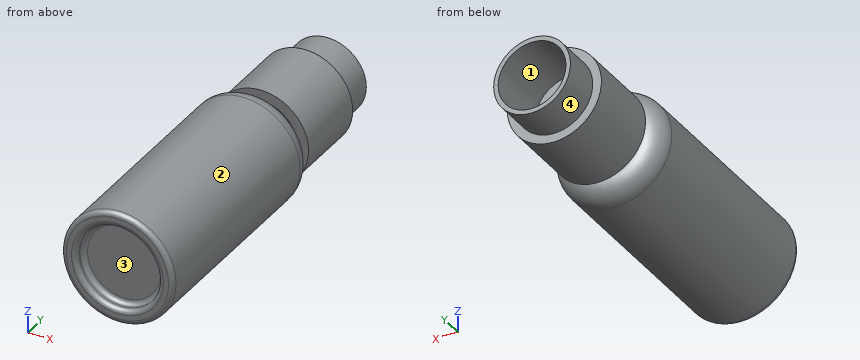
```python
from build123d import *


with BuildPart() as part:
    # Sketch1 → Revolve1 (revolve)
    with BuildSketch(Plane.XY):
        with BuildLine():
            ThreePointArc((8.75, 1), (9.042893219, 0.292893219), (9.75, 0))
            Line((9.75, 0), (10.875, 0))
            ThreePointArc((10.875, 0), (11.582106781, 0.292893219), (11.875, 1))
            Line((11.875, 1), (11.875, 46.5))
            ThreePointArc((11.875, 46.5), (10.593592168, 49.593592168), (7.5, 50.875))
            Line((7.5, 50.875), (7.75, 50.875))
            Line((7.75, 50.875), (7.75, 52.875))
            Line((7.75, 52.875), (10, 52.875))
            Line((10, 52.875), (10, 69.075))
            Line((10, 69.075), (8.15, 69.075))
            Line((8.15, 69.075), (8.15, 77.275))
            Line((8.15, 77.275), (7.2, 77.275))
            Line((7.2, 77.275), (7.2, 63.575))
            Line((7.2, 63.575), (0, 63.575))
            Line((0, 63.575), (0, 2.409558552))
            Line((0, 2.409558552), (7.75, 2.409558552))
            ThreePointArc((7.75, 2.409558552), (8.457106781, 2.116665333), (8.75, 1.409558552))
            Line((8.75, 1.409558552), (8.75, 1))
        make_face()
    revolve(axis=Axis((0, 65.8, 0), (0, -1, 0)))


solid = part.part
```
Geometry: final body of the model. Coordinates: model frame, mm. Face numbers are marked on the shaded views. A direction names the side the tool comes from. Coordinates: 2 decimals unless noted, no trailing zeros. Order: outer loops, then holes, each group sorted by start corner. A loop starts at its lowest first (then second) coordinate and runs counter-clockwise, first axis right, second up. Notation, with made-up numbers: M 9.25,45 L 26.25,45 A17 ccw 26.25,71 Z; hole C -14.75,12 d4. An arc over 180 degrees is marked long. Answer in a Markdown table with one row per item. Add a question column.
Q1. Reachability of the marked faces 1 and 2 from +Z, -Z, +X, -X, +Y, -Y: full face, straight path, thin tool, end or side. Return the list, or none.
Q2. Section query C-C on y = 18. Return the cut outline in (x, z) (3 decimals).
Q3. Mould query, pull axis X, two halves, no side actions, for the marked faces 3 and 4. Classes: released by +X, released by -X, zero draft, split by the parting line, or undercut.
Q4. Contact query for flat-ended pins moving along their axis: P1, Ø6, axis at x = -4.5, z = -4, coming from the -Y side; P2, Ø4, axis at x = 6, y = 45, coming from the +Z side; P3, Ø4, axis at x = 7, y = 14, coming from the -Z side. Output: stop coordinate, or through.
Q5. Line query: L1, parallel to Z at x = 0, y = 70.25; L2, parallel to Z at x = 0.25, y = 6.5; L3, parallel to Y at x = 4.25, z = -8.75 (3 decimals). Output: solid intervals per line, ascending.
Completed:
| question | item | result |
|---|---|---|
| 1 | face 1 | +Y |
| 1 | face 2 | +Y, -Y |
| 2 | outline | C 0,0 d23.75 |
| 3 | face 3 | undercut |
| 3 | face 4 | split by the parting line |
| 4 | P1 | stops at y = 0.32 |
| 4 | P2 | stops at z = 11.18 |
| 4 | P3 | stops at z = -10.77 |
| 5 | L1 | z = -8.15 to -7.2, 7.2 to 8.15 |
| 5 | L2 | z = -11.87 to 11.87 |
| 5 | L3 | y = 0 to 50.265, 52.875 to 69.075 |
